The listing builds one solid part. Answer for the finished solid, in the listing's coordinates (mm). A direction names the side the tool comes from. Round coordinates to 2 decimals unless told otherwise and drop trailing zeros. Write each loop counter-clockwise with the first axis right and the second up, starting at its lowest first coordinate (ties: lowest second). Pieces come first, ordered by that corner, then holes. Notation, with made-up numbers: (-3, 8) - (2, 8) arc R18 cw to (2, 25) - close; hole circle Ø8 at (23.25, -1). An arc over 180 degrees is marked (long way). Answer in a Markdown table with one row per item.
Autodesk Inventor part; units mm, degrees
ref_plane "YZ Plane" through (0, 0, 0) normal (1, 0, 0) x (0, 1, 0)
ref_plane "XZ Plane" through (0, 0, 0) normal (0, 1, 0) x (-1, 0, 0)
ref_plane "XY Plane" through (0, 0, 0) normal (0, 0, 1) x (1, 0, 0)
sketch "Sketch1" plane through (0, 0, 0) normal (0, 0, 1) x (1, 0, 0)
  line L0 (0, 0) -> (12, 0) construction
  line L1 (12, 0) -> (12, 25)
  line L2 (12, 25) -> (0, 25) construction
  line L3 (0, 25) -> (0, 0)
  arc A0 (12, 25) -> (0, 25) centre (6, 25) ccw
  arc A1 (0, 0) -> (12, 0) centre (6, 0) ccw
  circle A2 centre (6, 0) radius 4
  circle A3 centre (6, 20) radius 4
  line L4 (0, 25) -> (12, 25)
  line L5 (12, 25) -> (12, 31)
  line L6 (12, 31) -> (0, 31)
  line L7 (0, 31) -> (0, 25)
  dimension "d0" = 12
  dimension "d1" = 25
  dimension "d3" = 8
  dimension "d16" = 8
  dimension "d17" = 20
extrude "Extrusion1" add sketch "Sketch1" along normal blind 13
sketch "Sketch2" plane through (12, 0, 0) normal (1, 0, 0) x (0, 0, -1)
  circle A0 centre (-6.5, 27) radius 1.5
  circle A1 centre (-6.5, 9) radius 1.5
  line L0 (0, 0) -> (-13, 0)
  point P0 (-6.5, 0)
  dimension "d6" = 3
  dimension "d7" = 3
  dimension "d8" = 18
  dimension "d9" = 9
extrude "Extrusion2" cut sketch "Sketch2" against normal through all
sketch "Sketch3" plane through (0, 0, 0) normal (-1, 0, 0) x (0, 0, 1)
  circle A0 centre (6.5, 27) radius 1.5
  circle A1 centre (6.5, 9) radius 1.5
  circle A2 centre (6.5, 27) radius 3
  circle A3 centre (6.5, 9) radius 3
  point P0 (0, 0)
  dimension "d12" = 6
  dimension "d13" = 6
extrude "Extrusion3" cut sketch "Sketch3" against normal blind 3
fillet "Fillet1" radius 1 2 edges at (0, 31, 6.5) (12, 31, 6.5)
properties part number "z axis arm3"
(1) Section D-D (x = 9.25) is taken. Give the vertices of the cut face in (y, z), and give its area (3 significant figures).
Checked values:
| item | result |
|---|---|
| outline | (-5.04, 0) - (-2.33, 0) - (-2.33, 13) - (-5.04, 13) - close; (2.33, 0) - (17.67, 0) - (17.67, 13) - (2.33, 13) - close; (22.33, 0) - (31, 0) - (31, 13) - (22.33, 13) - close; hole circle Ø3 at (9, 6.5); hole circle Ø3 at (27, 6.5) |
| area | 333 mm2 |
(2) Find the intervals of material crossed by line 1 (Y direction, x = 6, z = 4.25); line 2 (Y direction, x = 1.75, z = 6.5); line 3 (Y direction, x = 5.5, z = 6.25), in increasing order.
Checked values:
| item | result |
|---|---|
| line 1 | y = -6 to -4, 4 to 16, 24 to 31 |
| line 2 | y = -4.24 to 6, 12 to 24, 30 to 31 |
| line 3 | y = -5.98 to -3.97, 3.97 to 7.52, 10.48 to 16.03, 23.97 to 25.52, 28.48 to 31 |
(3) Section C-C (z = 6.5) is taken. State how many separate pieces and enclosed holes the cut face has, and give its area (3 significant figures).
Checked values:
| item | result |
|---|---|
| separate pieces | 3 |
| enclosed holes | 2 |
| area | 238 mm2 |
(4) For faces 4 (the flat face through (6, 31, 6)), 5 (the cylindrical face through (1.48, 25.85, 9.27)), determine the directions among +Z, -Z, +X, -X, +Y, -Y from which every point of the face is accessible in a straight line to the end or side of a thin tool.
Checked values:
| item | result |
|---|---|
| face 4 | +Z, -Z, +X, -X, +Y |
| face 5 | -X |
(5) Section A-A (x = 6) is taken. Give the vertices of the cut face in (y, z), and give its area (3 significant figures).
Checked values:
| item | result |
|---|---|
| outline | (-6, 0) - (-4, 0) - (-4, 13) - (-6, 13) - close; (4, 0) - (16, 0) - (16, 13) - (4, 13) - close; (24, 0) - (31, 0) - (31, 13) - (24, 13) - close; hole circle Ø3 at (9, 6.5); hole circle Ø3 at (27, 6.5) |
| area | 259 mm2 |
(6) For a pull along Z with two mould halves and no side action, classify faces 1 (the flat face through (6, 13, 0)), 2 (the flat face through (6, 13, 13)), 3 (the cylindrical face through (7.563, 28.487, 6.695)) as pulls with the +Z half, pulls with the -Z half, needs draft (parallel to the pull), parting line crosses it, or undercut.
Checked values:
| item | result |
|---|---|
| face 1 | pulls with the -Z half |
| face 2 | pulls with the +Z half |
| face 3 | undercut |
(7) Section B-B (y = 9) is taken. Give the vertices of the cut face in (x, z).
Checked values:
| item | result |
|---|---|
| outline | (0, 0) - (12, 0) - (12, 5) - (3, 5) - (3, 3.5) - (0, 3.5) - close; (0, 9.5) - (3, 9.5) - (3, 8) - (12, 8) - (12, 13) - (0, 13) - close |
(8) Flat-ended cylindrical pins translate along their axes: pin 1 (2 mm diameter, centred on x = 6.5, y = 9, fed in from -Z); pin 2 (1.8 mm diameter, centred on y = 28, z = 7.5, fed in from -X); pin 3 (4 mm diameter, centred on x = 3.5, z = 4.5, fed in from -Y). Find the tip coordinate at first contact, or state that the pin passes through.
Checked values:
| item | result |
|---|---|
| pin 1 | stops at z = 0 |
| pin 2 | stops at x = 3 |
| pin 3 | stops at y = -5.98 |
